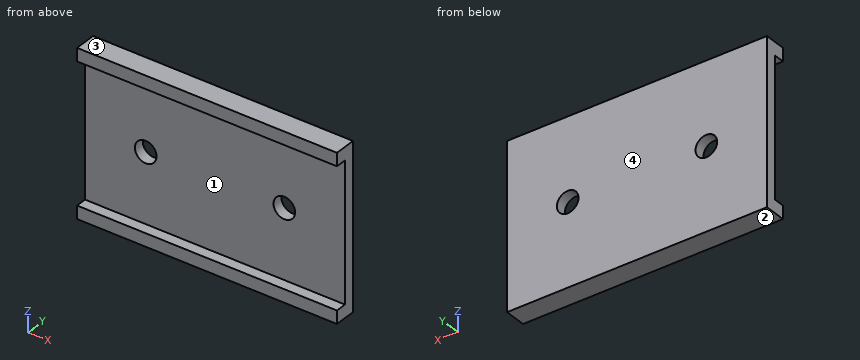
from build123d import *

# Parameters (mm, degrees)
F0_W     = 38.1
F0_H     = 19.05
F1_DEPTH = 1.5875
F2_R     = 1.5875
F3_DEPTH = 1.5885
F4_W     = 38.1
F4_H     = 2.54
F5_DEPTH = 1.5875
F6_W     = 38.1
F6_H     = 0.635
F7_DEPTH = 1.5875
F8_W     = 38.1
F8_H     = 0.635
F9_DEPTH = 1.5875


with BuildPart() as f1:
    # F0 (on Front) → F1 (new body)
    with BuildSketch(Plane.XZ):
        Rectangle(F0_W, F0_H)
    extrude(amount=F1_DEPTH)

    # F2 (on face) → F3 (cut, through all)
    with BuildSketch(Plane.XZ.offset(1.5875)):
        with Locations((-10.16, 0)):
            Circle(F2_R)
        with Locations((10.16, 0)):
            Circle(F2_R)
    extrude(amount=-F3_DEPTH, mode=Mode.SUBTRACT)

    # F4 (on face) → F5 (join, symmetric)
    with BuildSketch(Plane.XZ.offset(1.5875)):
        with Locations((0, -10.795)):
            Rectangle(F4_W, F4_H)
        with Locations((0, 10.795)):
            Rectangle(F4_W, F4_H)
    extrude(amount=F5_DEPTH, both=True)

    # F6 (on face) → F7 (cut)
    with BuildSketch(Plane.XZ.offset(3.175)):
        with Locations((0, 9.8425)):
            Rectangle(F6_W, F6_H)
    extrude(amount=-F7_DEPTH, mode=Mode.SUBTRACT)

    # F8 (on face) → F9 (cut)
    with BuildSketch(Plane.XZ.offset(3.175)):
        with Locations((0, -9.8425)):
            Rectangle(F8_W, F8_H)
    extrude(amount=-F9_DEPTH, mode=Mode.SUBTRACT)


solid = f1.part
Check sheet for the modelled part. Datum: model origin and axes. Units: mm. Face numbers are marked on the shaded views. Give positions to 0.01 mm unless a question says otherwise; leave off trailing zeros. Loops run counter-clockwise (first coordinate to the right, second up) from the corner with the lowest first, then second, coordinate; pieces in that order, holes last. Notation, with made-up numbers: M -26,84.25 L -16,84.25 A15 cw -16,102.25 Z; hole C 21.5,62.25 d10. An arc over 180 degrees is marked long. Use a Markdown table: item, result. Add a question column.
Q1. Scan lines: line 1 along Z through (x, y) = (-10.16, -1.1) (1 decimal); line 2 along Z through (x, y) = (-10, -2.15) (3 decimals); line 3 along X through (y, z) = (-1.15, -0.5). Record each from-to range of solid material in increasing order. Write a range as [from, to].
Q2. Sectioned sample at B-B, the plane z = 0. Record the cut outline in (x, y).
Q3. Sectioned sample at A-A, the plane x = 10.16. Record the cut outline in (y, z) (1 decimal).
Q4. Sectioned sample at D-D, the plane x = -15. Record the cut outline in (y, z) (1 decimal).
Q5. Go/stop test with flat-tipped pins: pin 1 (12 mm diameter, centred on x = -10, z = 2, fed in from -Y); pin 2 (1.9 mm diameter, centred on x = 10.16, z = 0, fed in from +Y). Record where each tip stops, or that it passes through.
Q6. Sectioned sample at C-C, the plane y = -2.7. Record the cut outline in (x, z) (3 decimals), then the cut area to 3 significant figures.
Q7. Mould release check, pull along Z, two halves, no side actions. Record for the marked faces 1, 2, 3 and 4: pulls with the +Z half, pulls with the -Z half, needs draft (parallel to the pull), parting line crosses it, or undercut.
Verdict:
| question | item | result |
|---|---|---|
| 1 | line 1 | [-12.1, -1.6], [1.6, 12.1] |
| 1 | line 2 | [-12.065, -10.16], [10.16, 12.065] |
| 1 | line 3 | [-19.05, -11.67], [-8.65, 8.65], [11.67, 19.05] |
| 2 | outline | M -19.05,-1.59 L -11.75,-1.59 L -11.75,0 L -19.05,0 Z; M -8.57,-1.59 L 8.57,-1.59 L 8.57,0 L -8.57,0 Z; M 11.75,-1.59 L 19.05,-1.59 L 19.05,0 L 11.75,0 Z |
| 3 | outline | M -3.2,-12.1 L 0,-12.1 L 0,-1.6 L -1.6,-1.6 L -1.6,-10.2 L -3.2,-10.2 Z; M -3.2,10.2 L -1.6,10.2 L -1.6,1.6 L 0,1.6 L 0,12.1 L -3.2,12.1 Z |
| 4 | outline | M -3.2,-12.1 L 0,-12.1 L 0,12.1 L -3.2,12.1 L -3.2,10.2 L -1.6,10.2 L -1.6,-10.2 L -3.2,-10.2 Z |
| 5 | pin 1 | y = -1.59 |
| 5 | pin 2 | through |
| 6 | outline | M -19.05,-12.065 L 19.05,-12.065 L 19.05,-10.16 L -19.05,-10.16 Z; M -19.05,10.16 L 19.05,10.16 L 19.05,12.065 L -19.05,12.065 Z |
| 6 | area | 145 mm^2 |
| 7 | face 1 | undercut |
| 7 | face 2 | pulls with the -Z half |
| 7 | face 3 | pulls with the +Z half |
| 7 | face 4 | needs draft |
